Input: part model. Units: mm. Frame: model coordinates. A direction names the side the tool comes from. Give positions to 0.01 mm unless a question says otherwise; leave off trailing zeros. Write each loop counter-clockwise with the first axis right and the second up, starting at its lowest first coordinate (ties: lowest second). Pieces come first, ordered by that corner, then holes. Notation, with made-up numbers: (71, 4) -> (80, 4) arc R22 ccw to (80, 21) -> close; hole circle Ø5 at (71.5, 12.5). An arc over 180 degrees is marked (long way). Return JSON: item names as keys, results as strings. Group by question number.
Item 1: Pin query (flat end, axial travel): P1, Ø1.4, axis at y = -4, z = -76, coming from the -X side; P2, Ø1, axis at x = 21, y = -1, coming from the +Z side; P3, Ø3, axis at y = -4, z = 0.5, coming from the +X side; P4, Ø2.5, axis at x = 15.5, z = -56.05, coming from the +Y side. Return the tip coordinate at first contact, or that it passes through.
Item 2: Mould query, pull axis X, two halves, no side actions, for faces 5 (the face through (1, -3, 20.4)), 6 (the face through (-22, -3, -93)), 7 (the face through (15, -3, -69.799)). Classes: released by +X, released by -X, zero draft, split by the parting line, or undercut.
Item 3: Section D-D, the plane z = -15.5. Return loops of the section in (x, y).
Item 4: Section B-B, the plane x = 0. Return loops of the section in (y, z) (3 decimals), then the cut area to 3 significant figures.
Item 5: Line query: line 1 (X direction, y = -0.15, z = -34.5); line 2 (X direction, y = -0.45, z = 20); line 3 (X direction, y = -1.2, z = -69.5) (3 decimals). Output: solid intervals per line, ascending. Write a range as [from, to].
Item 6: Set-up query: faces 1 (the face through (-20, -3, -69.799)), 2 (the face through (13.354, -3, -72)), 3 (the face through (25, -3, -90.602)), 4 (the face through (6.35, -3, 22)). Return all of +Z, -Z, +X, -X, +Y, -Y with unobstructed straight access to the full face (end or side cutting, diameter ignored); none if empty.
Item 7: Section C-C, the plane x = 10. Return loops of the section in (y, z) (3 decimals).
Item 8: Section A-A, the plane z = 0. Return loops of the section in (x, y).
from build123d import *

# Parameters (mm, degrees)
F0_R     = 1.5
F0_R_2   = 11.5
F0_R_3   = 2
F0_W     = 12.7
F0_H     = 5.842
F0_R_4   = 7.7
F1_DEPTH = 5.842
F2_R     = 3.175
F4_DEPTH = 5.843
F5_R     = 2.0828
F6_DEPTH = 25.4


with BuildPart() as f1:
    # F0 (on Front) → F1 (new body)
    with BuildSketch(Plane.XZ):
        Polygon((22, 28.575), (-22, 28.575), (-22, -52.5018), (-27.842, -52.5018), (-27.842, -65.2018), (-22, -65.2018), (-22, -77.9018), (-27.842, -77.9018), (-27.842, -90.6018), (-22, -90.6018), (-22, -95.25), (22, -95.25), (22, -90.6018), (27.842, -90.6018), (27.842, -77.9018), (22, -77.9018), (22, -65.2018), (27.842, -65.2018), (27.842, -52.5018), (22, -52.5018), align=None)
        with Locations((-15.5, -87.0518)):
            Circle(F0_R, mode=Mode.SUBTRACT)
        with Locations((-15.5, -56.0518)):
            Circle(F0_R, mode=Mode.SUBTRACT)
        with Locations((0, -71.5518)):
            Circle(F0_R_2, mode=Mode.SUBTRACT)
        with Locations((15.5, -87.0518)):
            Circle(F0_R, mode=Mode.SUBTRACT)
        with Locations((15.5, -56.0518)):
            Circle(F0_R, mode=Mode.SUBTRACT)
        with Locations((-14.062533, -33.3375)):
            Circle(F0_R_3, mode=Mode.SUBTRACT)
        with Locations((-12.7, 22.225)):
            Rectangle(F0_W, F0_H, mode=Mode.SUBTRACT)
        with Locations((14.062533, -33.3375)):
            Circle(F0_R_3, mode=Mode.SUBTRACT)
        Circle(F0_R_4, mode=Mode.SUBTRACT)
        with Locations((12.7, 22.225)):
            Rectangle(F0_W, F0_H, mode=Mode.SUBTRACT)
    extrude(amount=F1_DEPTH)

    # F2
    f2_edges = [f1.edges().sort_by_distance(p)[0] for p in [
        (-22, -2.921, 28.575),
        (22, -2.921, 28.575),
    ]]
    fillet(f2_edges, radius=F2_R)

    # F3 (on face) → F4 (cut, through all)
    with BuildSketch(Plane.XZ.offset(5.842)):
        Polygon((-18.825, -69.7992), (-22, -69.7992), (-22, -73.3044), (-18.825, -73.3044), (-18.825, -75.52055), (-15.846875, -75.52055), (-15.846875, -73.3044), (-13.3545, -73.3044), (-13.3545, -69.7992), (-15.846875, -69.7992), (-15.846875, -67.58305), (-18.825, -67.58305), align=None)
        Polygon((22, -73.3044), (22, -69.7992), (18.825, -69.7992), (18.825, -67.58305), (15.846875, -67.58305), (15.846875, -69.7992), (13.3545, -69.7992), (13.3545, -73.3044), (15.846875, -73.3044), (15.846875, -75.52055), (18.825, -75.52055), (18.825, -73.3044), align=None)
    extrude(amount=-F4_DEPTH, mode=Mode.SUBTRACT)

    # F5 (on face) → F6 (cut)
    with BuildSketch(Plane.XZ.offset(5.842)):
        with Locations((0, 22.225)):
            Circle(F5_R)
    extrude(amount=-F6_DEPTH, mode=Mode.SUBTRACT)


solid = f1.part
Answer below:
{
 "1": {"P1": "stops at x = -22", "P2": "stops at z = 28.1", "P3": "stops at x = 22", "P4": "passes through"},
 "2": {"face 5": "undercut", "face 6": "released by -X", "face 7": "zero draft"},
 "3": {"outline": "(-22, -5.84) -> (22, -5.84) -> (22, 0) -> (-22, 0) -> close"},
 "4": {"outline": "(-5.842, -95.25) -> (0, -95.25) -> (0, -83.052) -> (-5.842, -83.052) -> close; (-5.842, -60.052) -> (0, -60.052) -> (0, -7.7) -> (-5.842, -7.7) -> close; (-5.842, 7.7) -> (0, 7.7) -> (0, 20.142) -> (-5.842, 20.142) -> close; (-5.842, 24.308) -> (0, 24.308) -> (0, 28.575) -> (-5.842, 28.575) -> close", "area": "475 mm2"},
 "5": {"line 1": "x = [-22, -15.69], [-12.44, 12.44], [15.69, 22]", "line 2": "x = [-22, -19.05], [-6.35, 6.35], [19.05, 22]", "line 3": "x = [-22, -18.825], [-15.847, -11.315], [11.315, 15.847], [18.825, 22]"},
 "6": {"face 1": "-X, +Y, -Y", "face 2": "+X, +Y, -Y", "face 3": "-Z, +X, +Y, -Y", "face 4": "+Y, -Y"},
 "7": {"outline": "(-5.842, -95.25) -> (0, -95.25) -> (0, -77.231) -> (-5.842, -77.231) -> close; (-5.842, -65.873) -> (0, -65.873) -> (0, 19.304) -> (-5.842, 19.304) -> close; (-5.842, 25.146) -> (0, 25.146) -> (0, 28.575) -> (-5.842, 28.575) -> close"},
 "8": {"outline": "(-22, -5.84) -> (-7.7, -5.84) -> (-7.7, 0) -> (-22, 0) -> close; (7.7, -5.84) -> (22, -5.84) -> (22, 0) -> (7.7, 0) -> close"}
}
